CAD build for the part. Positions are in the model's coordinates, mm. A direction names the side the tool comes from. Round coordinates to 2 decimals unless told otherwise and drop trailing zeros. Loops run counter-clockwise (first coordinate to the right, second up) from the corner with the lowest first, then second, coordinate; pieces in that order, holes last.
Autodesk Inventor part; units mm, degrees
ref_plane "YZ Plane" through (0, 0, 0) normal (1, 0, 0) x (0, 1, 0)
ref_plane "XZ Plane" through (0, 0, 0) normal (0, 1, 0) x (-1, 0, 0)
ref_plane "XY Plane" through (0, 0, 0) normal (0, 0, 1) x (1, 0, 0)
sketch "Эскиз2" plane through (0, 0, 0) normal (1, 0, 0) x (0, 1, 0)
  line L0 (0, 0) -> (20, 0)
  line L1 (20, 0) -> (20, 20)
  line L2 (20, 20) -> (0, 20)
  line L3 (0, 20) -> (0, 0)
  line L4 (18.5, 18.5) -> (1.5, 18.5)
  line L5 (1.5, 18.5) -> (1.5, 1.5)
  line L6 (1.5, 1.5) -> (18.5, 1.5)
  line L7 (18.5, 1.5) -> (18.5, 18.5)
  point P0 (10, 18.5)
  point P1 (10, 20)
  point P2 (18.5, 10)
  point P3 (20, 10)
  dimension "d0" = 20
  dimension "d1" = 1.5
extrude "Выдавливание1" add sketch "Эскиз2" along normal blind 90
sketch "Эскиз3" plane through (0, 0, 20) normal (0, 0, 1) x (1, 0, 0)
  circle A0 centre (6, 10) radius 2
  circle A1 centre (84, 10) radius 2
  line L0 (90, 20) -> (90, 0)
  line L1 (0, 20) -> (0, 0)
  point P0 (90, 10)
  point P1 (0, 10)
  point P2 (90, 10)
  point P3 (0, 10)
  dimension "d6" = 6
  dimension "d7" = 6
  dimension "d10" = 4
extrude "Выдавливание2" cut sketch "Эскиз3" against normal through all
properties part number "section"
Item 1: Cut at D-D, the plane x = 84. Give the cut face in (y, z), plus the area to 3 significant figures.
Answers follow:
outline: (0, 0) - (8, 0) - (8, 1.5) - (1.5, 1.5) - (1.5, 18.5) - (8, 18.5) - (8, 20) - (0, 20) - close; (12, 0) - (20, 0) - (20, 20) - (12, 20) - (12, 18.5) - (18.5, 18.5) - (18.5, 1.5) - (12, 1.5) - close
area: 99.0 mm2
Item 2: Probe line 1 (Y direction, x = 16, z = 9.75); line 2 (Y direction, x = 84, z = 18.9). List the from-to ranges inside material, lowest first.
Answers follow:
line 1: y = 0 to 1.5, 18.5 to 20
line 2: y = 0 to 8, 12 to 20
Item 3: Flat gauge pin, fed straight in: P1, Ø2.5, axis at x = 6, y = 10, coming from the +Z side. Where does the tip first touch, or does it go through?
Answers follow:
P1: passes through
Item 4: Cut at C-C, the plane z = 14.75. Give the cut face in (x, y), plus the area to 3 significant figures.
Answers follow:
outline: (0, 0) - (90, 0) - (90, 1.5) - (0, 1.5) - close; (0, 18.5) - (90, 18.5) - (90, 20) - (0, 20) - close
area: 270 mm2
Item 5: 3-axis set-ups, long thin cutter, end or side, ignore diameter. For faces 4 (the cylindrical face through (6, 12, 19)), 5 (the flat face through (44, 10, 18.5)): which of +Z, -Z, +X, -X, +Y, -Y reach the whole face in a straight line?
Answers follow:
face 4: +Z, -Z
face 5: +X, -X
Item 6: Cut at A-A, the plane y = 10. Give the cut face in (x, z), plus the area to 3 significant figures.
Answers follow:
outline: (0, 0) - (4, 0) - (4, 1.5) - (0, 1.5) - close; (0, 18.5) - (4, 18.5) - (4, 20) - (0, 20) - close; (8, 0) - (82, 0) - (82, 1.5) - (8, 1.5) - close; (8, 18.5) - (82, 18.5) - (82, 20) - (8, 20) - close; (86, 0) - (90, 0) - (90, 1.5) - (86, 1.5) - close; (86, 18.5) - (90, 18.5) - (90, 20) - (86, 20) - close
area: 246 mm2
Item 7: Two-plate mould, pull along Z, no slides. Class faces 1 (the flat face through (44, 10, 0)), 2 (the flat face through (44, 18.5, 10)), 3 (the cylindrical face through (85.908, 10.601, 19.26)): released by +Z, released by -Z, zero draft, split by the parting line, or undercut.
Answers follow:
face 1: released by -Z
face 2: undercut
face 3: zero draft
Item 8: Cut at B-B, the plane x = 44. Give the cut face in (y, z).
Answers follow:
outline: (0, 0) - (20, 0) - (20, 20) - (0, 20) - close; hole (1.5, 1.5) - (18.5, 1.5) - (18.5, 18.5) - (1.5, 18.5) - close
